Model file for the job. Use its own axes, mm. Round coordinates to 2 decimals unless told otherwise and drop trailing zeros. Write each loop counter-clockwise with the first axis right and the second up, starting at its lowest first coordinate (ties: lowest second). Pieces come first, ordered by that corner, then holes. Notation, with made-up numbers: (-9.75, 67.5) - (38.25, 67.5) arc R20 cw to (38.25, 91.5) - close; hole circle Ø3 at (31, 20.5). An arc over 180 degrees is marked (long way). Answer as a JSON object with one key per item and string values. Group by question number.
Autodesk Inventor part; units mm, degrees
ref_plane "YZ Plane" through (0, 0, 0) normal (1, 0, 0) x (0, 1, 0)
ref_plane "XZ Plane" through (0, 0, 0) normal (0, 1, 0) x (-1, 0, 0)
ref_plane "XY Plane" through (0, 0, 0) normal (0, 0, 1) x (1, 0, 0)
sketch "Sketch1" plane through (0, 0, 0) normal (0, 1, 0) x (-1, 0, 0)
  line L0 (0, 0) -> (80, 0)
  line L1 (80, 0) -> (80, -25)
  line L2 (80, -25) -> (0, -25)
  line L3 (0, -25) -> (0, 0)
  dimension "d0" = 80
  dimension "d1" = 25
extrude "Extrusion1" add sketch "Sketch1" along normal blind 100
fillet "Fillet1" radius 40 2 edges at (0, 100, -12.5) (-80, 100, -12.5)
sketch "Sketch2" plane through (0, 0, -25) normal (0, 0, -1) x (-1, 0, 0)
  arc A0 (80, 60) -> (0, 60) centre (40, 60) ccw
  circle A1 centre (40, 60) radius 2.5
  point P0 (0, 0)
  dimension "d5" = 5
extrude "Extrusion2" cut sketch "Sketch2" against normal blind 100
properties part number "Foot"
(1) Slice it at B-B (x = -55). Write the cut outline in (y, z), then the cut area to 3 significant figures.
(2) Slice it at C-C (y = 90). Write the cut outline in (x, z), then the cut area to 3 significant figures.
(3) Pull direction X, two halves, no side cores. Call faces 1 (the cylindrical face through (-42.31, 59.04, -12.68)), 2 (the flat face through (0, 30, -13)), 3 (the flat face through (-39, 49, 0)): pulls with the +X half, pulls with the -X half, needs draft (parallel to the pull), parting line crosses it, or undercut.
(4) Flat gauge pin, fed straight in: pin 1 (3 mm diameter, centred on y = 67, z = -21, fed in from +X). Where does the tip first touch, or does it go through?
(5) Drill centre lines: line 1 (Y direction, x = -40, z = -19); line 2 (Y direction, x = -54.5, z = -9.5); line 3 (Y direction, x = -74, z = -9.25). Where is each one in solid material? Low to high. Write a range as from..to.
Answer:
{
 "1": {"outline": "(0, -25) - (97.08, -25) - (97.08, 0) - (0, 0) - close", "area": "2,430 mm²"},
 "2": {"outline": "(-66.46, -25) - (-13.54, -25) - (-13.54, 0) - (-66.46, 0) - close", "area": "1,320 mm²"},
 "3": {"face 1": "undercut", "face 2": "pulls with the +X half", "face 3": "needs draft"},
 "4": {"pin 1": "x = -0.38"},
 "5": {"line 1": "0..57.5, 62.5..100", "line 2": "0..97.28", "line 3": "0..81.07"}
}
